from build123d import *

# Parameters (mm, degrees)
BOSS_EXTRUDE1_DEPTH = 4
DRAFT1_ANGLE        = -45
DRAFT2_ANGLE        = -30.5
CUT_EXTRUDE5_DEPTH  = 2
CUT_EXTRUDE6_DEPTH  = 212.923325802
CUT_EXTRUDE9_DEPTH  = 2.2
CUT_EXTRUDE7_DEPTH  = 8.686291501
CUT_EXTRUDE8_DEPTH  = 8.686291501
CUT_EXTRUDE10_DEPTH = 2.2


with BuildPart() as part:
    # Sketch1 → Boss-Extrude1 (new body)
    with BuildSketch(Plane(origin=(0, 0, 0), x_dir=(1, 0, 0), z_dir=(0, 1, 0))):
        Polygon((52.494351143, -151.133854852), (51.789004581, -165.258389755), (104.862009772, -177.770248363), (115.348319519, -168.281449289), (108.186209242, -114.225971655), (94.061674339, -113.520625094), align=None)
    extrude(amount=BOSS_EXTRUDE1_DEPTH)

    # Draft1
    draft1_faces = [part.faces().sort_by_distance(p)[0] for p in [
        (73.278012741, 2, 132.327239973),
        (110.105164645, 2, 173.025848826),
        (52.141677862, 2, 158.196122303),
        (101.12394179, 2, 113.873298375),
    ]]
    draft(draft1_faces, Plane(origin=(0, 0, 0), x_dir=(0, 0, -1), z_dir=(0, -1, 0)), DRAFT1_ANGLE)

    # Draft2
    draft2_faces = [part.faces().sort_by_distance(p)[0] for p in [
        (78.138469796, 1.940570555, 171.470225357),
        (111.74202401, 1.940570555, 141.063210709),
    ]]
    draft(draft2_faces, Plane(origin=(0, 0, 0), x_dir=(0, 0, -1), z_dir=(0, -1, 0)), DRAFT2_ANGLE)

    # Sketch2 → Cut-Extrude5 (cut)
    with BuildSketch(Plane.XZ):
        Polygon((75.849733352, 144.111731538), (97.991394115, 168.581035955), (106.889322994, 160.52952295), (84.747662231, 136.060218533), align=None)
    extrude(amount=-CUT_EXTRUDE5_DEPTH, mode=Mode.SUBTRACT)

    # Sketch3 → Cut-Extrude6 (cut, through all)
    with BuildSketch(Plane.XZ.offset(-2)):
        Polygon((95.139816593, 165.429686144), (97.735045849, 163.081328184), (100.586623371, 166.232677995), (104.294093738, 162.87788091), (101.442516215, 159.726531099), (104.037745471, 157.378173139), (87.599239753, 139.211568345), (78.701310874, 147.263081349), align=None)
    extrude(amount=-CUT_EXTRUDE6_DEPTH, mode=Mode.SUBTRACT)

    # Sketch7 → Cut-Extrude9 (cut, along a direction that is not the sketch's normal)
    with BuildSketch(Plane(origin=(67.825186868, 101.086869254, 74.955314434), x_dir=(-0.5807891989379262, -0.19614622185114675, 0.7900699754139267), z_dir=(0.4744399537114777, 0.7071067811865489, 0.5243154873949929))):
        Polygon((74.094551817, 123.420131254), (69.290768622, 124.80709449), (69.845553917, 126.728607768), (74.649337111, 125.341644532), align=None)
    extrude(amount=-CUT_EXTRUDE9_DEPTH, dir=(0.6709594170704366, 0, 0.7414940732362599), mode=Mode.SUBTRACT)

    # Sketch4 → Cut-Extrude7 (cut, along a direction that is not the sketch's normal)
    with BuildSketch(Plane(origin=(0, 4, 0), x_dir=(1, 0, 0), z_dir=(0, 1, 0))):
        Polygon((112.587766826, -165.384890501), (111.435934245, -166.427154957), (111.53570927, -157.444566839), align=None)
    extrude(amount=-CUT_EXTRUDE7_DEPTH, dir=(-0.6637345426247422, 0.6785983445458476, -0.3145802659200979), mode=Mode.SUBTRACT)

    # Sketch6 → Cut-Extrude8 (cut, along a direction that is not the sketch's normal)
    with BuildSketch(Plane(origin=(0, 4, 0), x_dir=(1, 0, 0), z_dir=(0, 1, 0))):
        Polygon((102.254887128, -174.734854565), (103.406719709, -173.692590108), (94.458880925, -172.896961139), align=None)
    extrude(amount=-CUT_EXTRUDE8_DEPTH, dir=(-0.24688935673809265, 0.6785983445458336, -0.6917730352573054), mode=Mode.SUBTRACT)

    # Sketch8 → Cut-Extrude10 (cut, along a direction that is not the sketch's normal)
    with BuildSketch(Plane(origin=(29.94613408, -29.98345025, 1.495440583), x_dir=(0.7079857233236485, 0.7053499867326429, -0.03517970702195721), z_dir=(-0.7062267451533468, 0.7071067811865487, -0.03526732808291803))):
        Polygon((34.993140865, -160.762185663), (35.345376313, -155.774608076), (33.350345278, -155.633713897), (32.99810983, -160.621291484), align=None)
    cut_extrude10 = extrude(amount=-CUT_EXTRUDE10_DEPTH, dir=(-0.9987554411064721, 0, -0.04987553368352402), mode=Mode.SUBTRACT)

    # Mirror1: Cut-Extrude10 across plane
    add(cut_extrude10.mirror(Plane(origin=(-25.545209091, 0, 23.115219958), x_dir=(0.6709594170704504, 0, 0.7414940732362473), z_dir=(-0.7414940732362473, 0, 0.6709594170704505))), mode=Mode.SUBTRACT)


solid = part.part
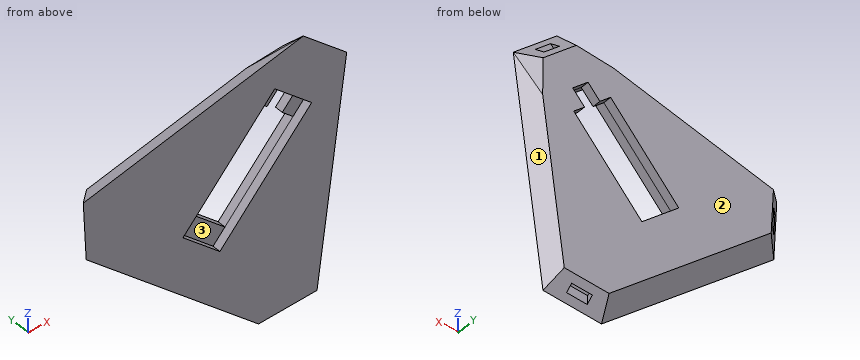
Model file for the job. Use its own axes, mm. Face numbers are marked on the shaded views. Round coordinates to 2 decimals unless told otherwise and drop trailing zeros. Order: outer loops, then holes, each group sorted by start corner. A loop starts at its lowest first (then second) coordinate and runs counter-clockwise, first axis right, second up. Notation, with made-up numbers: M 71,-36.5 L 130,-36.5 A22 cw 130,-30.5 Z; hole C 14.25,-1.5 d11. An arc over 180 degrees is marked long. Write each question's results on one line, items separated by ' | '. Start each with the question number.
(1) Probe probe 1 along X at (y, z) = (2.9, 164); probe 2 along X at (y, z) = (0.3, 153); probe 3 along Z at (x, y) = (92.5, 1.2). List the from-to ranges inside material, lowest first. Write a range as from..to.
(2) Saw through at B-B, the plane y = 3.35. Give the cut face in (x, z).
(3) Saw through at C-C, the plane z = 162. Give the cut face in (x, y), then the cut area to 3 significant figures.
(4) Saw through at A-A, the plane x = 81. Give the cut face in (y, z).
(5) Drop flat-ended pins along their axis: pin 1 (0.7 mm diameter, centred on x = 101, z = 115.5, fed in from +Y); pin 2 (1.2 mm diameter, centred on x = 55, z = 157, fed in from +Y). Give the stop position or say it passes through.
(6) Two-plate mould, pull along Z, no slides. Class the marked faces 1, 2 and 3: pulls with the +Z half, pulls with the -Z half, needs draft (parallel to the pull), parting line crosses it, or undercut.
(7) Saw through at D-D, the plane x = 97. Give the cut face in (y, z), then the cut area to 3 significant figures.
Established:
1) probe 1: x = 54.76..93.85, 96.72..98.57, 103.05..112.54 | probe 2: x = 52.7..83.89, 100.08..113.15 | probe 3: z = 116.55..144.63, 162.51..174.13
2) outline: M 55.2,164.04 L 55.77,152.69 L 95.28,116.94 L 106.63,117.5 L 112.16,159.21 L 112.07,166.73 L 103.64,174.36 L 96.15,173.69 Z; hole M 78.7,147.26 L 87.6,139.21 L 104.04,157.38 L 101.44,159.73 L 104.29,162.88 L 100.59,166.23 L 97.74,163.08 L 95.14,165.43 Z
3) outline: M 51.95,0 L 92.04,0 L 92.04,4 L 55.96,4 Z; M 103.5,2 L 105.26,2 L 105.26,0 L 114.52,0 L 113.14,2.32 L 111.49,4 L 103.5,4 Z | area: 188 mm^2
4) outline: M 0,125.34 L 4,130.73 L 4,145.18 L 2,145.18 L 2,139.45 L 0,139.45 Z; M 0,149.8 L 4,149.8 L 4,169.72 L 0,172.14 Z
5) pin 1: stops at y = 1.29 | pin 2: stops at y = 3.4
6) face 1: pulls with the -Z half | face 2: needs draft | face 3: undercut
7) outline: M 0,113.67 L 4,117.67 L 4,149.6 L 0,149.6 Z; M 0,167.49 L 2,167.49 L 2,163.75 L 4,163.75 L 4,173.12 L 3.02,174.09 L 0,175.92 Z | area: 172 mm^2
